The listing builds one solid part. Answer for the finished solid, in the listing's coordinates (mm). Coordinates: 2 decimals unless noted, no trailing zeros. Order: outer loops, then holes, each group sorted by start corner. A loop starts at its lowest first (then second) coordinate and runs counter-clockwise, first axis right, second up. Notation, with made-up numbers: (28.25, -22) - (75.25, -22) arc R17 cw to (75.25, -12) - close; hole circle Ø5 at (-22.5, 28). An arc over 180 degrees is marked (long way). Use a Markdown table: item, result. Add a question column.
Item 1: The part is cut by section B-B, the plane y = -6. Give the vertices of the cut face in (x, z), then the cut area to 3 significant figures.
Item 2: The part is cut by section D-D, the plane z = 7.25. Give the vertices of the cut face in (x, y), then the cut area to 3 significant figures.
Item 3: Find the intervals of material crossed by line 1 along Z through (x, y) = (0, -3); line 2 along Y through (x, z) = (4, -7); line 3 along Y through (x, z) = (2, -5.25), in increasing order.
Item 4: The part is cut by section C-C, the plane x = -4.5. Give the vertices of the cut face in (y, z).
Item 5: Flat-ended cylindrical pins translate along their axes: P1, Ø1, axis at x = 3.5, y = -10, coming from the -Z side; P2, Ø1, axis at y = -20.5, z = 6.5, coming from the -X side; P3, Ø12, axis at x = -7.5, y = -20, coming from the -Z side. Find the tip coordinate at first contact, or state that the pin passes through.
Item 6: The mould has two halves that part along Z. Classify faces 1 (the cylindrical face through (-0.596, -6.084, -2.685)), 2 (the flat face through (0, -25, 0)), 3 (the cylindrical face through (-1.302, -12.325, 9.915)), 4 (the cylindrical face through (-0.1, -12.4, -4.5)): released by +Z, released by -Z, zero draft, split by the parting line, or undercut.
Item 7: The part is cut by section A-A, the plane z = -5.5. Give the vertices of the cut face in (x, y), then the cut area to 3 significant figures.
from build123d import *

# Parameters (mm, degrees)
F0_R          = 10
F1_DEPTH      = 25
F2_R          = 7.5
F3_DEPTH      = 10.001
F3_DEPTH_BACK = 10.001
F5_D          = 5.5
F5_DEPTH      = 12
F5_TIP        = 1.6523667023


with BuildPart() as f1:
    # F0 (on Front) → F1 (new body)
    with BuildSketch(Plane.XZ):
        Circle(F0_R)
    extrude(amount=F1_DEPTH)

    # F2 (on Right) → F3 (cut, two sides)
    with BuildSketch(Plane.YZ) as f3_sk:
        with Locations((-12.5, -12)):
            Circle(F2_R)
    extrude(amount=F3_DEPTH, mode=Mode.SUBTRACT)
    extrude(f3_sk.sketch, amount=-F3_DEPTH_BACK, mode=Mode.SUBTRACT)

    # F5
    with Locations(Plane(origin=(0, 0, 0), x_dir=(-1, 0, 0), z_dir=(0, 1, 0))):
        with Locations((0, 0)):
            Hole(F5_D / 2, depth=F5_DEPTH)
            with Locations((0, 0, -(F5_DEPTH + F5_TIP / 2))):  # 118° drill point
                Cone(0, F5_D / 2, F5_TIP, mode=Mode.SUBTRACT)


solid = f1.part
Solution:
| question | item | result |
|---|---|---|
| 1 | outline | (-5.64, -8.26) - (5.64, -8.26) arc R10 ccw (long way) to start; hole circle Ø5.5 at (0, 0) |
| 1 | area | 277 mm2 |
| 2 | outline | (-6.89, -25) - (6.89, -25) - (6.89, 0) - (-6.89, 0) - close |
| 2 | area | 344 mm2 |
| 3 | line 1 | z = -10 to -2.75, 2.75 to 10 |
| 3 | line 2 | y = -25 to -18.09, -6.91 to 0 |
| 3 | line 3 | y = -25 to -15.77, -9.23 to 0 |
| 4 | outline | (-25, -8.93) - (-19.34, -8.93) arc R7.5 cw to (-5.66, -8.93) - (0, -8.93) - (0, 8.93) - (-25, 8.93) - close |
| 5 | P1 | stops at z = -5.13 |
| 5 | P2 | stops at x = -8 |
| 5 | P3 | stops at z = -9.89 |
| 6 | face 1 | undercut |
| 6 | face 2 | zero draft |
| 6 | face 3 | split by the parting line |
| 6 | face 4 | released by -Z |
| 7 | outline | (-8.35, -25) - (8.35, -25) - (8.35, -16.24) - (-8.35, -16.24) - close; (-8.35, -8.76) - (8.35, -8.76) - (8.35, 0) - (-8.35, 0) - close |
| 7 | area | 293 mm2 |
